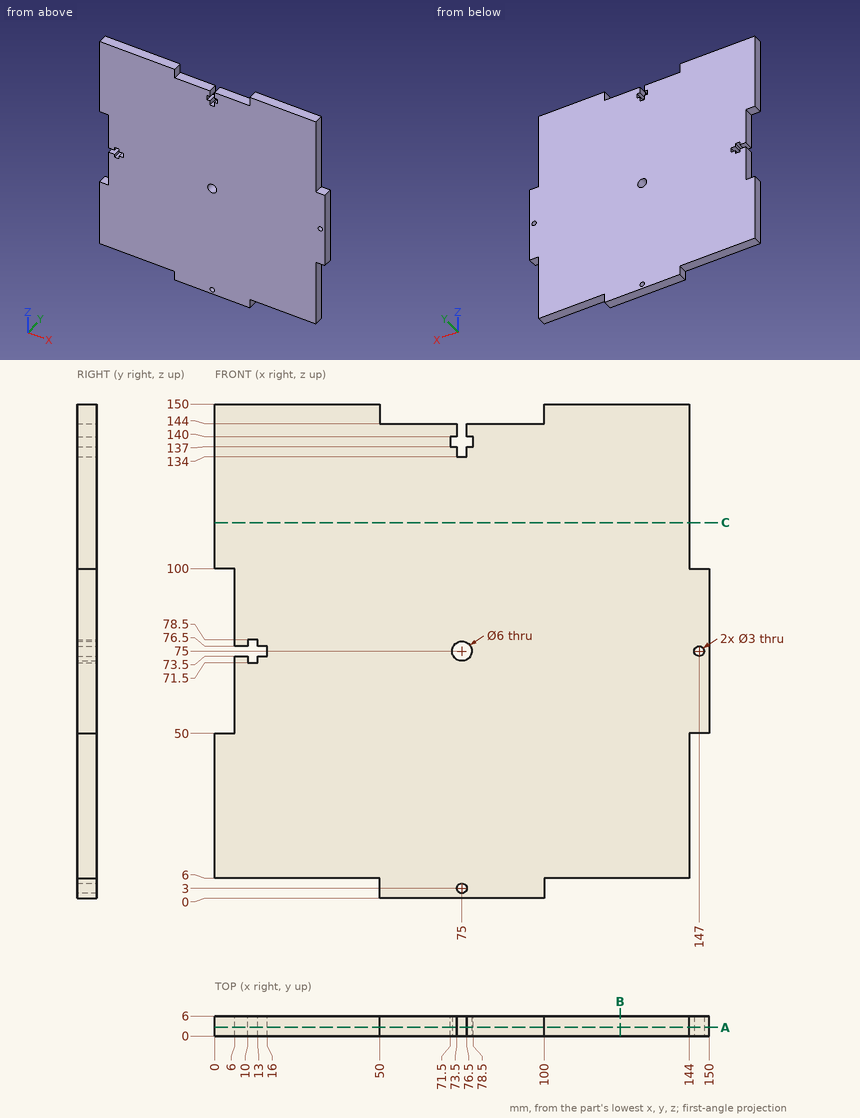
The drawing under review shows one solid part. Ordinate dimensions are in mm from its lowest x, y, z. Coordinates: 2 decimals unless noted, no trailing zeros. Order: outer loops, then holes, each group sorted by start corner. A loop starts at its lowest first (then second) coordinate and runs counter-clockwise, first axis right, second up. Notation, with made-up numbers: (36, 10) -> (69, 10) arc R32 cw to (69, 49) -> close; hole circle Ø10 at (61, -13.75). An arc over 180 degrees is marked (long way). One line per item, written item: value.
1) We need section B-B, the plane x = 123. Give the boundary of the cut face in (y, z).
Output values:
outline: (0, 6) -> (6, 6) -> (6, 150) -> (0, 150) -> close
2) We need section A-A, the plane y = 2.6. Count the separate pieces of the cut face and the enclosed holes in it, then the cut area to 3 significant figures.
Output values:
separate pieces: 1
enclosed holes: 3
area: 20,600 mm2
3) To check wall thickness, follow probe 1 along X at (y, z) = (4.75, 75); probe 2 along Z at (x, y) = (147, 4.6). State the ranges of each line that lie inside material, in increasing order. Write a range as [from, to].
Output values:
probe 1: x = [16, 72], [78, 145.5], [148.5, 150]
probe 2: z = [50, 73.5], [76.5, 100]
4) We need section C-C, the plane z = 114. Give the boundary of the cut face in (x, y), then the cut area to 3 significant figures.
Output values:
outline: (0, 0) -> (144, 0) -> (144, 6) -> (0, 6) -> close
area: 864 mm2
5) Clearance check with flat-ended pins moving along their axes: P1, Ø5, axis at x = 75, z = 75, coming from the +Y side; P2, Ø1.8, axis at y = 1.5, z = 146, coming from the +X side; P3, Ø3, axis at x = 104, y = 3, coming from the -Z side; P4, Ø1.8, axis at y = 2.5, z = 2, coming from the -X side. State where each tip first meets the part, or that it passes through.
Output values:
P1: passes through
P2: stops at x = 144
P3: stops at z = 6
P4: stops at x = 50
